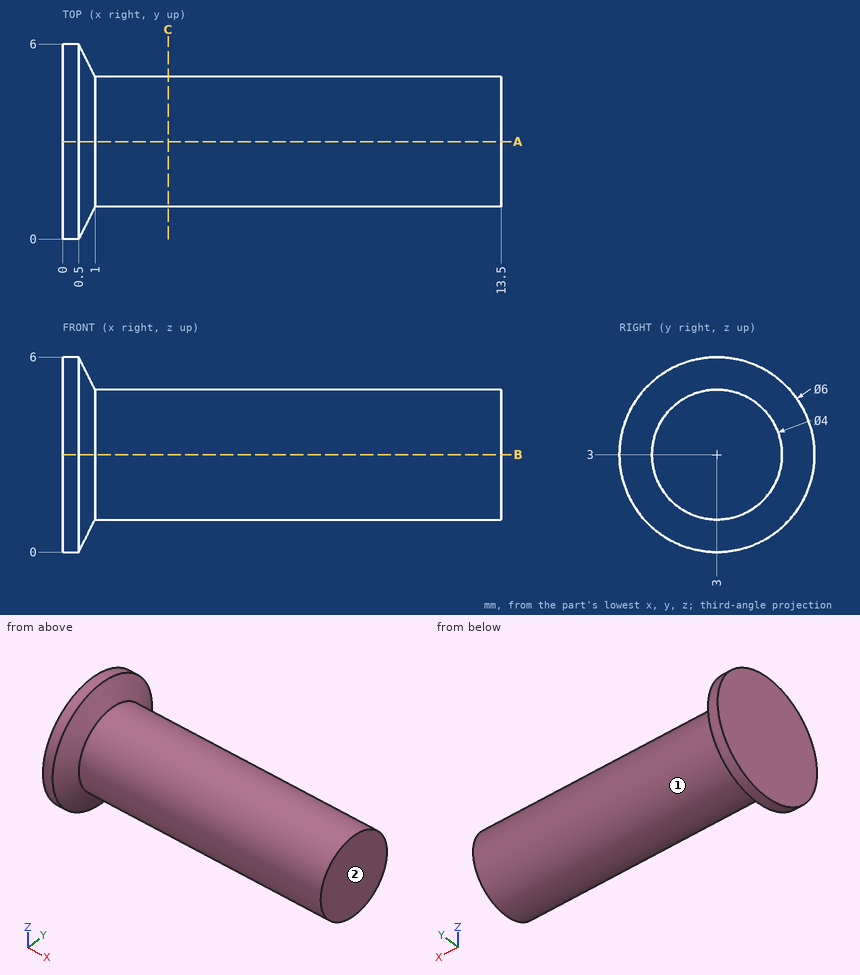
Can you work these out from the drawing? Everything is in mm from the part's minimum corner. A direction names the side the tool comes from. Give positions to 0.01 mm unless a question says otherwise; leave off trailing zeros. Order: outer loops, then holes, each group sorted by start corner. A loop starts at its lowest first (then second) coordinate and runs counter-clockwise, first axis right, second up.
1. Suppose I cut it at C-C (x = 3.25). List the corners of the cut face in (y, z) for me, plus the area to 3 significant figures.
2. Suppose I cut it at A-A (y = 3). List the corners of the cut face in (x, z) for me.
3. For the marked faces 1 and 2, which set-ups out of +Z, -Z, +X, -X, +Y, -Y let a thin tool reach every point of the face, with its end or its side?
4. I need wall thicknesses on L1, parallel to Z at x = 11.25, y = 2.9; L2, parallel to X at y = 1.8, z = 0.4. Which ranges of each line are inside material? Lowest first, please.
5. Will these pins go through, and if not, where does the flat tip stop? P1, Ø2, axis at y = 0.5, z = 3.5, coming from the -X side; P2, Ø2, axis at x = 1.5, z = 1.5, coming from the -Y side; P3, Ø1.5, axis at x = 12, z = 4, coming from the +Y side.
Solved:
1. outline: circle Ø4 at (3, 3)
1. area: 12.6 mm2
2. outline: (0, 0) - (0.5, 0) - (1, 1) - (13.5, 1) - (13.5, 5) - (1, 5) - (0.5, 6) - (0, 6) - close
3. face 1: +X
3. face 2: +Z, -Z, +X, +Y, -Y
4. L1: z = 1 to 5
4. L2: x = 0 to 0.57
5. P1: stops at x = 0
5. P2: stops at y = 0.34
5. P3: stops at y = 4.98
